from build123d import *

# Parameters (mm, degrees)
SKETCH1_R            = 11
SKETCH1_R_2          = 8
SKETCH1_W            = 45.13
SKETCH1_H            = 7
BOSS_EXTRUDE1_DEPTH  = 10
SKETCH2_W            = 1.71
SKETCH2_H            = 4
CUT_EXTRUDE1_DEPTH   = 10
SKETCH3_W            = 20
SKETCH3_H            = 10
BOSS_EXTRUDE2_DEPTH  = 3
CUT_EXTRUDE2_START   = -3
CUT_EXTRUDE2_DEPTH   = 3
SKETCH6_W            = 20
SKETCH6_H            = 7
BOSS_EXTRUDE3_DEPTH  = 2
SKETCH7_R            = 1.5
CUT_EXTRUDE5_DEPTH   = 44
SKETCH9_W            = 1.71
SKETCH9_H            = 7
BOSS_EXTRUDE4_DEPTH  = 3
CUT_EXTRUDE6_START   = -1
SKETCH11_R           = 8
CUT_EXTRUDE6_DEPTH   = 1
BOSS_EXTRUDE6_DEPTH  = 1
BOSS_EXTRUDE7_START  = 6
SKETCH13_R           = 8
BOSS_EXTRUDE7_DEPTH  = 6
SKETCH14_R           = 8
BOSS_EXTRUDE8_DEPTH  = 40
SKETCH15_R           = 7.5
BOSS_EXTRUDE9_DEPTH  = 30
BOSS_EXTRUDE10_START = 6.5
BOSS_EXTRUDE10_DEPTH = 6.5
SKETCH17_R           = 15.773418916
SKETCH17_R_2         = 7
CUT_EXTRUDE7_DEPTH   = 30
SKETCH18_R           = 7.1
BOSS_EXTRUDE11_DEPTH = 30
SKETCH19_R           = 7.2
BOSS_EXTRUDE12_DEPTH = 30
SKETCH20_R           = 12.810748173
SKETCH20_R_2         = 7.15
CUT_EXTRUDE8_DEPTH   = 30
SKETCH21_R           = 7.15
CUT_EXTRUDE9_DEPTH   = 10
SKETCH22_R           = 8
SKETCH22_R_2         = 7.15
CUT_EXTRUDE10_DEPTH  = 10
SKETCH25_W           = 1.71
SKETCH25_H           = 3
SKETCH25_W_2         = 20
CUT_EXTRUDE13_DEPTH  = 21
BOSS_EXTRUDE13_DEPTH = 20
BOSS_EXTRUDE14_START = -20
BOSS_EXTRUDE14_DEPTH = 20
SKETCH28_R           = 1.5
CUT_EXTRUDE14_DEPTH  = 50
SKETCH29_W           = 45.13
SKETCH29_H           = 13.5
BOSS_EXTRUDE15_DEPTH = 4
FILLET1_R            = 10
FILLET2_R            = 2


with BuildPart() as part:
    # Sketch1 → Boss-Extrude1 (new body)
    # profile 1 of 2: a face of its own
    with BuildSketch(Plane(origin=(0, 0, 0), x_dir=(1, 0, 0), z_dir=(0, 1, 0))):
        with Locations((22.565, -8)):
            Circle(SKETCH1_R)
        with Locations(Location((22.565, -8, 0), (0, 0, 270))):
            Circle(SKETCH1_R_2, mode=Mode.SUBTRACT)
    # profile 2 of 2: a face of its own
    with BuildSketch(Plane(origin=(0, 0, 0), x_dir=(1, 0, 0), z_dir=(0, 1, 0))):
        with Locations((22.565, 3.5)):
            Rectangle(SKETCH1_W, SKETCH1_H)
    extrude(amount=BOSS_EXTRUDE1_DEPTH)

    # Sketch2 → Cut-Extrude1 (cut)
    with BuildSketch(Plane(origin=(0, 10, 0), x_dir=(1, 0, 0), z_dir=(0, 1, 0))):
        with Locations((0.855, 5)):
            Rectangle(SKETCH2_W, SKETCH2_H)
        with Locations((22.565, 5)):
            Rectangle(SKETCH2_W, SKETCH2_H)
        with Locations((44.275, 5)):
            Rectangle(SKETCH2_W, SKETCH2_H)
    extrude(amount=-CUT_EXTRUDE1_DEPTH, mode=Mode.SUBTRACT)

    # Sketch3 → Boss-Extrude2 (add)
    with BuildSketch(Plane(origin=(0, 0, -7), x_dir=(-1, 0, 0), z_dir=(0, 0, -1))):
        with Locations((-33.42, 5)):
            Rectangle(SKETCH3_W, SKETCH3_H)
        with Locations((-11.71, 5)):
            Rectangle(SKETCH3_W, SKETCH3_H)
    extrude(amount=BOSS_EXTRUDE2_DEPTH)

    # Sketch4 → Cut-Extrude2 (cut)
    with BuildSketch(Plane(origin=(0, 10, 0), x_dir=(1, 0, 0), z_dir=(0, 1, 0)).offset(CUT_EXTRUDE2_START)):
        with BuildLine():
            Line((21.71, 3), (21.71, 10))
            Line((21.71, 10), (1.71, 10))
            Line((1.71, 10), (1.71, 3))
            Line((1.71, 3), (0, 3))
            Line((0, 3), (0, 0))
            Line((0, 0), (15.015165565, 0))
            ThreePointArc((15.015165565, 0), (22.565, -19), (30.114834435, 0))
            Line((30.114834435, 0), (45.13, 0))
            Line((45.13, 0), (45.13, 3))
            Line((45.13, 3), (43.42, 3))
            Line((43.42, 3), (43.42, 10))
            Line((43.42, 10), (23.42, 10))
            Line((23.42, 10), (23.42, 3))
            Line((23.42, 3), (21.71, 3))
        make_face()
    extrude(amount=CUT_EXTRUDE2_DEPTH, mode=Mode.SUBTRACT)

    # Sketch6 → Boss-Extrude3 (add)
    with BuildSketch(Plane(origin=(0, 0, -10), x_dir=(-1, 0, 0), z_dir=(0, 0, -1))):
        with Locations((-33.42, 3.5)):
            Rectangle(SKETCH6_W, SKETCH6_H)
        with Locations((-11.71, 3.5)):
            Rectangle(SKETCH6_W, SKETCH6_H)
    extrude(amount=BOSS_EXTRUDE3_DEPTH)

    # Sketch7 → Cut-Extrude5 (cut)
    with BuildSketch(Plane.ZY.offset(-1.71)):
        with Locations((-8.5, 3.5)):
            Circle(SKETCH7_R)
    extrude(amount=-CUT_EXTRUDE5_DEPTH, mode=Mode.SUBTRACT)

    # Sketch9 → Boss-Extrude4 (add)
    with BuildSketch(Plane(origin=(0, 0, -3), x_dir=(-1, 0, 0), z_dir=(0, 0, -1))):
        with Locations((-22.565, 3.5)):
            Rectangle(SKETCH9_W, SKETCH9_H)
        with Locations((-0.855, 3.5)):
            Rectangle(SKETCH9_W, SKETCH9_H)
        with Locations((-44.275, 3.5)):
            Rectangle(SKETCH9_W, SKETCH9_H)
    extrude(amount=BOSS_EXTRUDE4_DEPTH)

    # Sketch11 → Cut-Extrude6 (cut)
    with BuildSketch(Plane(origin=(0, 7, 0), x_dir=(1, 0, 0), z_dir=(0, 1, 0)).offset(CUT_EXTRUDE6_START)):
        with BuildLine():
            Line((45.13, 6), (43.42, 6))
            Line((43.42, 6), (43.42, 12))
            Line((43.42, 12), (23.42, 12))
            Line((23.42, 12), (23.42, 6))
            Line((23.42, 6), (21.71, 6))
            Line((21.71, 6), (21.71, 12))
            Line((21.71, 12), (1.71, 12))
            Line((1.71, 12), (1.71, 6))
            Line((1.71, 6), (0, 6))
            Line((0, 6), (0, 0))
            Line((0, 0), (15.015165565, 0))
            ThreePointArc((15.015165565, 0), (22.565, -19), (30.114834435, 0))
            Line((30.114834435, 0), (45.13, 0))
            Line((45.13, 0), (45.13, 6))
        make_face()
        with Locations(Location((22.565, -8, 0), (0, 0, 270))):
            Circle(SKETCH11_R, mode=Mode.SUBTRACT)
    extrude(amount=CUT_EXTRUDE6_DEPTH, mode=Mode.SUBTRACT)

    # Sketch12 → Boss-Extrude6 (add)
    with BuildSketch(Plane(origin=(0, 6, 0), x_dir=(1, 0, 0), z_dir=(0, 1, 0))):
        with BuildLine():
            Line((45.13, 0), (45.13, 6))
            Line((45.13, 6), (43.42, 6))
            Line((43.42, 6), (43.42, 12))
            Line((43.42, 12), (23.42, 12))
            Line((23.42, 12), (23.42, 6))
            Line((23.42, 6), (21.71, 6))
            Line((21.71, 6), (21.71, 12))
            Line((21.71, 12), (1.71, 12))
            Line((1.71, 12), (1.71, 6))
            Line((1.71, 6), (0, 6))
            Line((0, 6), (0, 0))
            Line((0, 0), (15.015165565, 0))
            ThreePointArc((15.015165565, 0), (22.565, -19), (30.114834435, 0))
            Line((30.114834435, 0), (45.13, 0))
        make_face()
    extrude(amount=BOSS_EXTRUDE6_DEPTH)

    # Sketch13 → Boss-Extrude7 (add)
    with BuildSketch(Plane.XZ.offset(-6).offset(BOSS_EXTRUDE7_START)):
        with Locations((22.565, 8)):
            Circle(SKETCH13_R)
    extrude(amount=-BOSS_EXTRUDE7_DEPTH)

    # Sketch14 → Boss-Extrude8 (add)
    with BuildSketch(Plane.XZ):
        with Locations(Location((22.565, 8, 0), (0, 0, 90))):
            Circle(SKETCH14_R)
    extrude(amount=BOSS_EXTRUDE8_DEPTH)

    # Sketch15 → Boss-Extrude9 (add)
    with BuildSketch(Plane.XZ.offset(40)):
        with Locations(Location((22.565, 8, 0), (0, 0, 270))):
            Circle(SKETCH15_R)
    extrude(amount=BOSS_EXTRUDE9_DEPTH)

    # Sketch16 → Boss-Extrude10 (add)
    with BuildSketch(Plane.XZ.offset(BOSS_EXTRUDE10_START)):
        with BuildLine():
            Line((43.42, -12), (43.42, -6))
            Line((43.42, -6), (45.13, -6))
            Line((45.13, -6), (45.13, 0))
            Line((45.13, 0), (30.114834435, 0))
            ThreePointArc((30.114834435, 0), (22.565, 19), (15.015165565, 0))
            Line((15.015165565, 0), (0, 0))
            Line((0, 0), (0, -6))
            Line((0, -6), (1.71, -6))
            Line((1.71, -6), (1.71, -12))
            Line((1.71, -12), (21.71, -12))
            Line((21.71, -12), (21.71, -6))
            Line((21.71, -6), (23.42, -6))
            Line((23.42, -6), (23.42, -12))
            Line((23.42, -12), (43.42, -12))
        make_face()
    extrude(amount=-BOSS_EXTRUDE10_DEPTH)

    # Sketch17 → Cut-Extrude7 (cut)
    with BuildSketch(Plane.XZ.offset(70)):
        with Locations((22.565, 8)):
            Circle(SKETCH17_R)
        with Locations(Location((22.565, 8, 0), (0, 0, 270))):
            Circle(SKETCH17_R_2, mode=Mode.SUBTRACT)
    extrude(amount=-CUT_EXTRUDE7_DEPTH, mode=Mode.SUBTRACT)

    # Sketch18 → Boss-Extrude11 (add)
    with BuildSketch(Plane.XZ.offset(70)):
        with Locations(Location((22.565, 8, 0), (0, 0, 270))):
            Circle(SKETCH18_R)
    extrude(amount=-BOSS_EXTRUDE11_DEPTH)

    # Sketch19 → Boss-Extrude12 (add)
    with BuildSketch(Plane.XZ.offset(70)):
        with Locations(Location((22.565, 8, 0), (0, 0, 270))):
            Circle(SKETCH19_R)
    extrude(amount=-BOSS_EXTRUDE12_DEPTH)

    # Sketch20 → Cut-Extrude8 (cut)
    with BuildSketch(Plane.XZ.offset(70)):
        with Locations((22.565, 8)):
            Circle(SKETCH20_R)
        with Locations(Location((22.565, 8, 0), (0, 0, 270))):
            Circle(SKETCH20_R_2, mode=Mode.SUBTRACT)
    extrude(amount=-CUT_EXTRUDE8_DEPTH, mode=Mode.SUBTRACT)

    # Sketch21 → Cut-Extrude9 (cut)
    with BuildSketch(Plane.XZ.offset(70)):
        with Locations(Location((22.565, 8, 0), (0, 0, 270))):
            Circle(SKETCH21_R)
    extrude(amount=-CUT_EXTRUDE9_DEPTH, mode=Mode.SUBTRACT)

    # Sketch22 → Cut-Extrude10 (cut)
    with BuildSketch(Plane.XZ.offset(40)):
        with Locations(Location((22.565, 8, 0), (0, 0, 270))):
            Circle(SKETCH22_R)
        with Locations(Location((22.565, 8, 0), (0, 0, 270))):
            Circle(SKETCH22_R_2, mode=Mode.SUBTRACT)
    extrude(amount=-CUT_EXTRUDE10_DEPTH, mode=Mode.SUBTRACT)

    # Sketch25 → Cut-Extrude13 (cut)
    with BuildSketch(Plane(origin=(0, 7, 0), x_dir=(1, 0, 0), z_dir=(0, 1, 0))):
        with Locations((0.855, 4.5)):
            Rectangle(SKETCH25_W, SKETCH25_H)
        with Locations((11.71, 10.5)):
            Rectangle(SKETCH25_W_2, SKETCH25_H)
        with Locations((33.42, 10.5)):
            Rectangle(SKETCH25_W_2, SKETCH25_H)
        with Locations((22.565, 4.5)):
            Rectangle(SKETCH25_W, SKETCH25_H)
        with Locations((44.275, 4.5)):
            Rectangle(SKETCH25_W, SKETCH25_H)
    extrude(amount=-CUT_EXTRUDE13_DEPTH, mode=Mode.SUBTRACT)

    # Sketch26 → Boss-Extrude13 (add)
    with BuildSketch(Plane.ZY.offset(-1.71)):
        with BuildLine():
            ThreePointArc((-7, 3.5), (-7.633974596, 4.724744871), (-9, 4.914213562))
            Line((-9, 4.914213562), (-9, 2.085786438))
            ThreePointArc((-9, 2.085786438), (-7.633974596, 2.275255129), (-7, 3.5))
        make_face()
    extrude(amount=-BOSS_EXTRUDE13_DEPTH)

    # Sketch27 → Boss-Extrude14 (add)
    with BuildSketch(Plane(origin=(43.42, 0, 0), x_dir=(0, 0, -1), z_dir=(1, 0, 0)).offset(BOSS_EXTRUDE14_START)):
        with BuildLine():
            Line((9, 2.085786438), (9, 4.914213562))
            ThreePointArc((9, 4.914213562), (7, 3.5), (9, 2.085786438))
        make_face()
    extrude(amount=BOSS_EXTRUDE14_DEPTH)

    # Sketch28 → Cut-Extrude14 (cut)
    with BuildSketch(Plane.ZY.offset(-1.71)):
        with Locations((-5.5, 3.5)):
            Circle(SKETCH28_R)
    extrude(amount=-CUT_EXTRUDE14_DEPTH, mode=Mode.SUBTRACT)

    # Sketch29 → Boss-Extrude15 (add)
    with BuildSketch(Plane.XY):
        with Locations((22.565, 0.25)):
            Rectangle(SKETCH29_W, SKETCH29_H)
    extrude(amount=BOSS_EXTRUDE15_DEPTH)

    # Fillet1
    fillet1_edges = [part.edges().sort_by_distance(p)[0] for p in [
        (32.811950766, 0.25, 4),
        (12.318049234, 0.25, 4),
    ]]
    fillet(fillet1_edges, radius=FILLET1_R)

    # Fillet2
    fillet2_edges = [part.edges().sort_by_distance(p)[0] for p in [
        (22.565, -6.5, 0),
    ]]
    fillet(fillet2_edges, radius=FILLET2_R)


solid = part.part
Part model, mm, in its own coordinate system. A direction names the side the tool comes from. Give positions to 0.01 mm unless a question says otherwise; leave off trailing zeros. Loops run counter-clockwise (first coordinate to the right, second up) from the corner with the lowest first, then second, coordinate; pieces in that order, holes last. Notation, with made-up numbers: M 34.25,9 L 52.25,9 A23 cw 52.25,17 Z; hole C -40,47 d11. An arc over 180 degrees is marked long. Put each result on its own line as item: value. Start each with the question number.
1) Pull direction Z, two halves, no side cores. Call faces 6 (the flat face through (33, 0, -9)), 7 (the cylindrical face through (33.28, 3.57, -7)), 8 (the flat face through (1, 0, 4)): +Z half, -Z half, draft (parallel to the pull), parting line (faces both ways), or undercut.
2) Saw through at B-B (y = 3.5). List the corners of the cut face in (x, z) (3 decimals), then the cut area to 3 significant figures.
3) Saw through at D-D (z = 8). List the corners of the cut face in (x, y) (3 decimals), then the cut area to 3 significant figures.
4) Probe probe 1 along Y at (x, z) = (33.5, -5.5); probe 2 along Y at (x, z) = (31, 2.25); probe 3 along X at (y, z) = (-1, -7). List the from-to ranges inside material, lowest first.
5) Saw through at C-C (x = 35). List the corners of the cut face in (y, z).
6) 3-axis set-ups, long thin cutter, end or side, ignore diameter. For faces 1 (the flat face through (44, 0, 4)), 2 (the flat face through (1.71, 0, -6)), 3 (the flat face through (18, -30, 14)), 4 (the flat face through (43.42, 0, -6)), 5 (the flat face through (23, 0, -3)): which of +Z, -Z, +X, -X, +Y, -Y reach the whole face in a straight line?
7) Saw through at A-A (z = -5.5). List the corners of the cut face in (x, y), then the cut area to 3 significant figures.
8) Flat gauge pins, fed straight in: pin 1 (1.8 mm diameter, centred on y = 3, z = -5.5, fed in from -X); pin 2 (1.9 mm diameter, centred on x = 44.5, y = 3, fed in from -Z); pin 3 (1.9 mm diameter, centred on x = 1, y = -2, fed in from -Z); pin 4 (0.7 mm diameter, centred on x = 1, y = 1, fed in from +Z). Where does each tip first touch, or does it go through?
Numbers:
1. face 6: -Z half
1. face 7: undercut
1. face 8: +Z half
2. outline: M 0,-3 L 1.71,-3 L 1.71,-4 L 21.71,-4 L 21.71,-3 L 23.42,-3 L 23.42,-4 L 43.42,-4 L 43.42,-3 L 45.13,-3 L 45.13,4 L 42.69,4 A10 cw 33.106,11.143 A11 ccw 12.024,11.143 A10 cw 2.44,4 L 0,4 Z; M 1.71,-9 L 21.71,-9 L 21.71,-7 L 1.71,-7 Z; M 23.42,-9 L 43.42,-9 L 43.42,-7 L 23.42,-7 Z
2. area: 745 mm^2
3. outline: M 10.44,-6.5 L 12.565,-6.5 A2 cw 14.565,-8.5 L 14.565,-30 L 15.415,-30 L 15.415,-60 L 29.715,-60 L 29.715,-30 L 30.565,-30 L 30.565,-8.5 A2 cw 32.565,-6.5 L 34.69,-6.5 L 34.69,7 L 10.44,7 Z
3. area: 1,130 mm^2
4. probe 1: -6.5 to 2, 5 to 7
4. probe 2: -6.5 to 7
4. probe 3: 1.71 to 21.71, 23.42 to 43.42
5. outline: M -6.5,-9 L 7,-9 L 7,7.61 L -6.5,7.61 Z; hole C 3.5,-5.5 d3
6. face 1: +Z, +X, +Y, -Y
6. face 2: -Z, -X, +Y, -Y
6. face 3: -Y
6. face 4: -Z, +X, +Y, -Y
6. face 5: -Z, +Y, -Y
7. outline: M 1.71,-6.5 L 21.71,-6.5 L 21.71,2 L 1.71,2 Z; M 1.71,5 L 21.71,5 L 21.71,7 L 1.71,7 Z; M 23.42,-6.5 L 43.42,-6.5 L 43.42,2 L 23.42,2 Z; M 23.42,5 L 43.42,5 L 43.42,7 L 23.42,7 Z
7. area: 420 mm^2
8. pin 1: through
8. pin 2: z = -3
8. pin 3: z = -9
8. pin 4: z = 4
